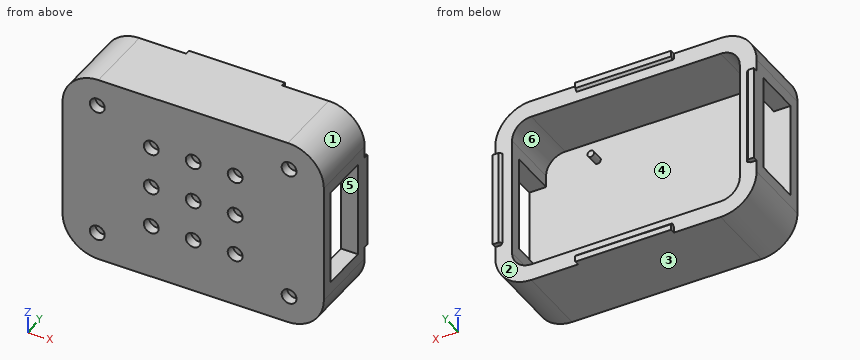
from build123d import *

# Parameters (mm, degrees)
BOSS_EXTRUDE1_DEPTH     = 5
SKETCH4_R               = 3.1
CUT_EXTRUDE1_DEPTH      = 4
BOSS_EXTRUDE3_DEPTH     = 30
CUT_EXTRUDE2_DEPTH      = 120.920807202
CUT_EXTRUDE2_DEPTH_BACK = 120.920807202
SKETCH7_W               = 40
SKETCH7_H               = 20
BOSS_EXTRUDE2_START     = 5
SKETCH3_R               = 1.35
BOSS_EXTRUDE2_DEPTH     = 5
BOSS_EXTRUDE6_DEPTH     = 20
BOSS_EXTRUDE7_DEPTH     = 20


with BuildPart() as part:
    # Sketch1 → Boss-Extrude1 (new body)
    with BuildSketch(Plane(origin=(0, 0, 0), x_dir=(1, 0, 0), z_dir=(0, 1, 0))):
        with BuildLine():
            Line((-39.5, 40), (39.5, 40))
            ThreePointArc((39.5, 40), (50.106601718, 35.606601718), (54.5, 25))
            Line((54.5, 25), (54.5, -25))
            ThreePointArc((54.5, -25), (50.106601718, -35.606601718), (39.5, -40))
            Line((39.5, -40), (-39.5, -40))
            ThreePointArc((-39.5, -40), (-50.106601718, -35.606601718), (-54.5, -25))
            Line((-54.5, -25), (-54.5, 25))
            ThreePointArc((-54.5, 25), (-50.106601718, 35.606601718), (-39.5, 40))
        make_face()
    extrude(amount=BOSS_EXTRUDE1_DEPTH)

    # Sketch4 → Cut-Extrude1 (cut)
    with BuildSketch(Plane(origin=(0, 0, 0), x_dir=(1, 0, 0), z_dir=(0, 1, 0))):
        with Locations(Location((-40, -28.424678982, 0), (0, 0, 270))):
            Circle(SKETCH4_R)
        with Locations(Location((40, -28.424678982, 0), (0, 0, 270))):
            Circle(SKETCH4_R)
        with Locations(Location((40, 28.424678982, 0), (0, 0, 270))):
            Circle(SKETCH4_R)
        with Locations(Location((-40, 28.424678982, 0), (0, 0, 270))):
            Circle(SKETCH4_R)
        with Locations(Location((-17.5, 0, 0), (0, 0, 270))):
            Circle(SKETCH4_R)
        with Locations(Location((0, -17.5, 0), (0, 0, 270))):
            Circle(SKETCH4_R)
        with Locations(Location((17.5, 0, 0), (0, 0, 270))):
            Circle(SKETCH4_R)
        with Locations(Location((0, 17.5, 0), (0, 0, 270))):
            Circle(SKETCH4_R)
        with Locations(Location((-17.5, 17.5, 0), (0, 0, 270))):
            Circle(SKETCH4_R)
        with Locations(Location((17.5, 17.5, 0), (0, 0, 270))):
            Circle(SKETCH4_R)
        with Locations(Location((17.5, -17.5, 0), (0, 0, 270))):
            Circle(SKETCH4_R)
        with Locations(Location((-17.5, -17.5, 0), (0, 0, 270))):
            Circle(SKETCH4_R)
        with Locations(Location((0, 0, 0), (0, 0, 270))):
            Circle(SKETCH4_R)
    extrude(amount=CUT_EXTRUDE1_DEPTH, mode=Mode.SUBTRACT)

    # Sketch1<3> → Boss-Extrude3 (add)
    with BuildSketch(Plane(origin=(0, 0, 0), x_dir=(1, 0, 0), z_dir=(0, 1, 0))):
        with BuildLine():
            Line((-39.5, 40), (39.5, 40))
            ThreePointArc((39.5, 40), (50.106601718, 35.606601718), (54.5, 25))
            Line((54.5, 25), (54.5, -25))
            ThreePointArc((54.5, -25), (50.106601718, -35.606601718), (39.5, -40))
            Line((39.5, -40), (-39.5, -40))
            ThreePointArc((-39.5, -40), (-50.106601718, -35.606601718), (-54.5, -25))
            Line((-54.5, -25), (-54.5, 25))
            ThreePointArc((-54.5, 25), (-50.106601718, 35.606601718), (-39.5, 40))
        make_face()
        with BuildLine():
            ThreePointArc((-39.5, 33), (-45.156854249, 30.656854249), (-47.5, 25))
            Line((-47.5, 25), (-47.5, -25))
            ThreePointArc((-47.5, -25), (-45.156854249, -30.656854249), (-39.5, -33))
            Line((-39.5, -33), (39.5, -33))
            ThreePointArc((39.5, -33), (45.156854249, -30.656854249), (47.5, -25))
            Line((47.5, -25), (47.5, 25))
            ThreePointArc((47.5, 25), (45.156854249, 30.656854249), (39.5, 33))
            Line((39.5, 33), (-39.5, 33))
        make_face(mode=Mode.SUBTRACT)
    extrude(amount=BOSS_EXTRUDE3_DEPTH)

    # Sketch7 → Cut-Extrude2 (cut, two sides: drawn at the far end of the back side and taken through both)
    with BuildSketch(Plane.ZY.offset(54.5).offset(-CUT_EXTRUDE2_DEPTH_BACK)):
        with Locations((0, 15)):
            Rectangle(SKETCH7_W, SKETCH7_H)
    extrude(amount=CUT_EXTRUDE2_DEPTH + CUT_EXTRUDE2_DEPTH_BACK, mode=Mode.SUBTRACT)

    # Sketch3 → Boss-Extrude2 (add)
    with BuildSketch(Plane(origin=(0, 0, 0), x_dir=(1, 0, 0), z_dir=(0, 1, 0)).offset(BOSS_EXTRUDE2_START)):
        with Locations(Location((26.04, 24.13, 0), (0, 0, 270))):
            Circle(SKETCH3_R)
        with Locations(Location((-40, 20.955, 0), (0, 0, 270))):
            Circle(SKETCH3_R)
        with Locations(Location((-40, -20.955, 0), (0, 0, 270))):
            Circle(SKETCH3_R)
        with Locations(Location((26.04, -24.13, 0), (0, 0, 270))):
            Circle(SKETCH3_R)
    extrude(amount=BOSS_EXTRUDE2_DEPTH)

    # Sketch10 → Boss-Extrude6 (add, symmetric)
    with BuildSketch(Plane(origin=(0, 0, 0), x_dir=(0, 0, -1), z_dir=(1, 0, 0))):
        Polygon((37.5, 30), (40, 30), (40, 32), (37.5, 32), (36.5, 31), align=None)
    boss_extrude6 = extrude(amount=BOSS_EXTRUDE6_DEPTH, both=True)

    # Mirror2: Boss-Extrude6 across plane
    add(boss_extrude6.mirror(Plane.XY))

    # Sketch12 → Boss-Extrude7 (add, symmetric)
    with BuildSketch(Plane.XY):
        Polygon((52, 30), (54.5, 30), (54.5, 32), (52, 32), (51, 31), align=None)
    boss_extrude7 = extrude(amount=BOSS_EXTRUDE7_DEPTH, both=True)

    # Mirror3: Boss-Extrude7 across plane
    add(boss_extrude7.mirror(Plane(origin=(0, 0, 0), x_dir=(0, 0, 1), z_dir=(1, 0, 0))))


solid = part.part
Read the model definition and answer for the solid it produces. Units are mm, in the model's axes. Face numbers are marked on the shaded views. A direction names the side the tool comes from. Give positions to 0.01 mm unless a question says otherwise; leave off trailing zeros. Write each loop counter-clockwise with the first axis right and the second up, starting at its lowest first coordinate (ties: lowest second). Pieces come first, ordered by that corner, then holes. Notation, with made-up numbers: (17, -31) -> (66, -31) arc R21 cw to (66, -6) -> close; hole circle Ø5 at (-17, -22.75). An arc over 180 degrees is marked (long way). Answer as a JSON object with one key per item and string values. Group by question number.
1) A tool of negligible diameter and unlimited length cuts with its end or side. For the marked faces 4, 5 and 6, from which of +Z, -Z, +X, -X, +Y, -Y can it reach the whole face along a straight path? Write none if from no direction.
2) Find section A-A (y = 16.5). Write down the section's boundary in (x, z).
3) The mould has two halves that part along X. Classify the marked faces 1, 2 and 3: +X half, -X half, draft (parallel to the pull), parting line (faces both ways), or undercut.
4) Find section D-D (z = -17.5). Count the separate pieces of the cut face and the enclosed holes in it, and give its area (3 significant figures).
5) Each of these flat-tipped pins is pushed along its axis until it touches: P1, Ø10, axis at x = -40, z = -28.42, coming from the -Y side; P2, Ø2, axis at y = 30.5, z = 39, coming from the +X side; P3, Ø0.8, axis at x = 25.5, z = 24, coming from the +Y side; P4, Ø4, axis at x = 43.5, y = 18.5, coming from the -Z side. Where does it stop, or does it pass through?
6) Find section B-B (z = 13). Write down the section's boundary in (x, y).
7) Find section C-C (x = -33.5). Write down the section's boundary in (y, z), and give its area (3 significant figures).
8) Consider L1, parallel to X at y = 2.8, z = 0; L2, parallel to Z at x = -13, y = 9; L3, parallel to Z at x = 17, y = 2. Determine where each line is inside the solid, lowest interval first. Write a range as from..to.
Values follow:
{
 "1": {"face 4": "none", "face 5": "+X, -X", "face 6": "+Y"},
 "2": {"outline": "(-54.5, -25) arc R15 ccw to (-39.5, -40) -> (39.5, -40) arc R15 ccw to (54.5, -25) -> (54.5, -20) -> (47.5, -20) -> (47.5, -25) arc R8 cw to (39.5, -33) -> (-39.5, -33) arc R8 cw to (-47.5, -25) -> (-47.5, -20) -> (-54.5, -20) -> close; (-54.5, 20) -> (-47.5, 20) -> (-47.5, 25) arc R8 cw to (-39.5, 33) -> (39.5, 33) arc R8 cw to (47.5, 25) -> (47.5, 20) -> (54.5, 20) -> (54.5, 25) arc R15 ccw to (39.5, 40) -> (-39.5, 40) arc R15 ccw to (-54.5, 25) -> close"},
 "3": {"face 1": "+X half", "face 2": "undercut", "face 3": "draft"},
 "4": {"separate pieces": "3", "enclosed holes": "0", "area": "553 mm2"},
 "5": {"P1": "stops at y = 0", "P2": "stops at x = 46.75", "P3": "stops at y = 10", "P4": "stops at z = -39.87"},
 "6": {"outline": "(-54.5, 0) -> (54.5, 0) -> (54.5, 5) -> (-54.5, 5) -> close; (-54.5, 25) -> (-47.5, 25) -> (-47.5, 30) -> (-52, 30) -> (-51, 31) -> (-52, 32) -> (-54.5, 32) -> close; (47.5, 25) -> (54.5, 25) -> (54.5, 32) -> (52, 32) -> (51, 31) -> (52, 30) -> (47.5, 30) -> close"},
 "7": {"outline": "(0, -40) -> (30, -40) -> (30, -33) -> (5, -33) -> (5, 33) -> (30, 33) -> (30, 40) -> (0, 40) -> close", "area": "750 mm2"},
 "8": {"L1": "x = -54.5..-20.6, -14.4..-3.1, 3.1..14.4, 20.6..54.5", "L2": "z = -40..-33, 33..40", "L3": "z = -40..-20.56, -14.44..-3.06, 3.06..14.44, 20.56..40"}
}
